```python
from build123d import *

# Parameters (mm, degrees)
SKETCH1_R                    = 33
BOSS_EXTRUDE1_DEPTH          = 3
CUT_EXTRUDE2_REACH           = 48.765
SKETCH3_R                    = 3.005
CUT_EXTRUDE3_REACH           = 48.765
CIRPATTERN2_COUNT            = 24
CUT_EXTRUDE1_REACH           = 48.68
SKETCH2_R                    = 1.5
CHAMFER1_SIZE                = 1.5
CIRPATTERN1_COUNT            = 6
CHAMFER1_OF_CIRPATTERN1_SIZE = 1.5
CUT_EXTRUDE4_REACH           = 48.68
SKETCH5_R                    = 1.5
CHAMFER2_SIZE                = 1.5
CIRPATTERN3_COUNT            = 6
CHAMFER2_OF_CIRPATTERN3_SIZE = 1.5


with BuildPart() as part:
    # Sketch1 → Boss-Extrude1 (new body)
    with BuildSketch(Plane(origin=(0, 0, 0), x_dir=(0, 0, -1), z_dir=(1, 0, 0))):
        Circle(SKETCH1_R)
    extrude(amount=BOSS_EXTRUDE1_DEPTH)

    # Sketch3 → Cut-Extrude2 (cut, up to next)
    with BuildSketch(Plane(origin=(3, 0, 0), x_dir=(0, 0, -1), z_dir=(1, 0, 0)), mode=Mode.PRIVATE) as cut_extrude2_sk1:
        Circle(SKETCH3_R)
    cut_extrude2_tool1 = extrude(cut_extrude2_sk1.sketch, amount=-CUT_EXTRUDE2_REACH, mode=Mode.PRIVATE) & part.part
    add(cut_extrude2_tool1.solids().sort_by_distance((3, 0, 0))[0], mode=Mode.SUBTRACT)

    # Sketch4 → Cut-Extrude3 (cut, up to next)
    with BuildSketch(Plane(origin=(3, 0, 0), x_dir=(0, 0, -1), z_dir=(1, 0, 0)), mode=Mode.PRIVATE) as cut_extrude3_sk1:
        with BuildLine():
            Line((-2, 33), (-2, 24.7))
            ThreePointArc((-2, 24.7), (0, 22.7), (2, 24.7))
            Line((2, 24.7), (2, 33))
            Line((2, 33), (-2, 33))
        make_face()
    cut_extrude3_tool1 = extrude(cut_extrude3_sk1.sketch, amount=-CUT_EXTRUDE3_REACH, mode=Mode.PRIVATE) & part.part
    cut_extrude3 = cut_extrude3_tool1.solids().sort_by_distance((3, 28.054508, 0))[0]
    add(cut_extrude3, mode=Mode.SUBTRACT)

    # CirPattern2: Cut-Extrude3 ×24 about axis
    cirpattern2_axis = Axis((0, 0, 0), (1, 0, 0))
    for i in range(1, CIRPATTERN2_COUNT):
        add(cut_extrude3.rotate(cirpattern2_axis, i * 360 / CIRPATTERN2_COUNT), mode=Mode.SUBTRACT)

    # Sketch2 → Cut-Extrude1 (cut, up to next)
    with BuildSketch(Plane(origin=(3, 0, 0), x_dir=(0, 0, -1), z_dir=(1, 0, 0)), mode=Mode.PRIVATE) as cut_extrude1_sk1:
        with Locations((2.610523844, 19.828897227)):
            Circle(SKETCH2_R)
    cut_extrude1_tool1 = extrude(cut_extrude1_sk1.sketch, amount=-CUT_EXTRUDE1_REACH, mode=Mode.PRIVATE) & part.part
    cut_extrude1 = cut_extrude1_tool1.solids().sort_by_distance((3, 19.828897, -2.610524))[0]
    add(cut_extrude1, mode=Mode.SUBTRACT)

    # Chamfer1
    chamfer1_edges = [part.edges().sort_by_distance(p)[0] for p in [
        (3, 19.828897227, -1.110523844),
    ]]
    chamfer(chamfer1_edges, length=CHAMFER1_SIZE)

    # CirPattern1: Cut-Extrude1 ×6 about axis
    cirpattern1_axis = Axis((0, 0, 0), (1, 0, 0))
    for i in range(1, CIRPATTERN1_COUNT):
        add(cut_extrude1.rotate(cirpattern1_axis, i * 360 / CIRPATTERN1_COUNT), mode=Mode.SUBTRACT)

    # Chamfer1 of CirPattern1
    chamfer1_of_cirpattern1_edges = [part.edges().sort_by_distance(p)[0] for p in [
        (3, 10.876190474, 16.617066806),
        (3, -8.952706753, 17.72759065),
        (3, -19.828897227, 1.110523844),
        (3, -10.876190474, -16.617066806),
        (3, 8.952706753, -17.72759065),
    ]]
    chamfer(chamfer1_of_cirpattern1_edges, length=CHAMFER1_OF_CIRPATTERN1_SIZE)

    # Sketch5 → Cut-Extrude4 (cut, up to next)
    with BuildSketch(Plane(origin=(3, 0, 0), x_dir=(0, 0, -1), z_dir=(1, 0, 0)), mode=Mode.PRIVATE) as cut_extrude4_sk1:
        with Locations((-3.635492607, 8.776855559)):
            Circle(SKETCH5_R)
    cut_extrude4_tool1 = extrude(cut_extrude4_sk1.sketch, amount=-CUT_EXTRUDE4_REACH, mode=Mode.PRIVATE) & part.part
    cut_extrude4 = cut_extrude4_tool1.solids().sort_by_distance((3, 8.776856, 3.635493))[0]
    add(cut_extrude4, mode=Mode.SUBTRACT)

    # Chamfer2
    chamfer2_edges = [part.edges().sort_by_distance(p)[0] for p in [
        (3, 8.776855559, 5.135492607),
    ]]
    chamfer(chamfer2_edges, length=CHAMFER2_SIZE)

    # CirPattern3: Cut-Extrude4 ×6 about axis
    cirpattern3_axis = Axis((0, 0, 0), (1, 0, 0))
    for i in range(1, CIRPATTERN3_COUNT):
        add(cut_extrude4.rotate(cirpattern3_axis, i * 360 / CIRPATTERN3_COUNT), mode=Mode.SUBTRACT)

    # Chamfer2 of CirPattern3
    chamfer2_of_cirpattern3_edges = [part.edges().sort_by_distance(p)[0] for p in [
        (3, -0.05903928, 10.168726183),
        (3, -8.835894838, 5.033233576),
        (3, -8.776855559, -5.135492607),
        (3, 0.05903928, -10.168726183),
        (3, 8.835894838, -5.033233576),
    ]]
    chamfer(chamfer2_of_cirpattern3_edges, length=CHAMFER2_OF_CIRPATTERN3_SIZE)


solid = part.part
```
Input: part model. Units: mm. Frame: model coordinates. A direction names the side the tool comes from. Round coordinates to 2 decimals unless told otherwise and drop trailing zeros. Answer as CSV lines item,"result".
1. Reachability of faces 5 (the cylindrical face through (1.5, -22.7, 0)), 6 (the flat face through (1.521, 27.376, 9.406)), 7 (the flat face through (1.52, 28.41, -5.54)) from +Z, -Z, +X, -X, +Y, -Y: full face, straight path, thin tool, end or side. Return the list, or none.
Geometry says:
face 5,"+X, -X, -Y"
face 6,"+X, -X, +Y"
face 7,"+X, -X"
2. Section A-A (x = 2.4). Give the number of separate pieces and of enclosed holes in the cut face, plus the area to 3 significant figures.
Geometry says:
separate pieces,"1"
enclosed holes,"13"
area,"2,230 mm^2"
3. Ray query, L1, parallel to Y at x = 2.15, z = 29.5; L2, parallel to Y at x = 0.65, z = 24.5; L3, parallel to Y at x = 0.6, z = -25. Return the intervals inside material, ascending. Write a range as [from, to].
Geometry says:
L1,"y = [-14.72, -9.98], [-5.83, -2], [2, 5.83], [9.98, 14.72]"
L2,"y = [-21.67, -16.45], [-11.84, -8.64], [-4.49, -1.99], [1.99, 4.49], [8.64, 11.84], [16.45, 21.67]"
L3,"y = [-21.54, -16.74], [-12.12, -8.77], [-4.63, -2], [2, 4.63], [8.77, 12.12], [16.74, 21.54]"
4. Mould query, pull axis Z, two halves, no side actions, for faces 1 (the cylindrical face through (1.479, 20.115, 26.161)), 2 (the cylindrical face through (0.76, -7.313, -3.961)), 3 (the flat face through (2, 2, 29)), 4 (the cylindrical face through (1.479, -26.2, -20.063)). Classes: +Z half, -Z half, draft (parallel to the pull), parting line (faces both ways), or undercut.
Geometry says:
face 1,"+Z half"
face 2,"undercut"
face 3,"draft"
face 4,"-Z half"
5. Contact query for flat-ended pins moving along their axis: P1, Ø1, axis at x = 1, y = 22, coming from the +Z side (3 decimals); P2, Ø5, axis at y = -7.54, z = 5.78, coming from the -X side; P3, Ø3.5, axis at y = 8.78, z = 3.64, coming from the +X side; P4, Ø1.5, axis at x = 1, z = -11.5, coming from the +Y side. Output: stop coordinate, or through.
Geometry says:
P1,"stops at z = 25.035"
P2,"stops at x = 0"
P3,"stops at x = 1.76"
P4,"stops at y = 31.2"
